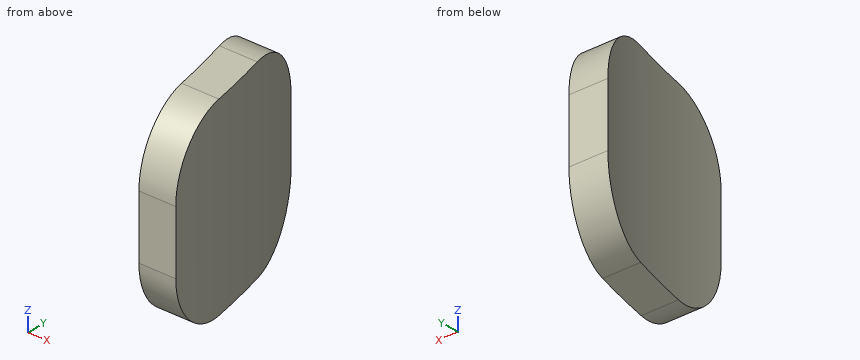
```python
from build123d import *

# Parameters (mm, degrees)
BOSS_EXTRUDE2_DEPTH     = 1066.8
CUT_EXTRUDE1_DEPTH      = 2806.00308884
CUT_EXTRUDE1_DEPTH_BACK = 2806.00308884


with BuildPart() as part:
    # Sketch1 → Boss-Extrude2 (new body)
    with BuildSketch(Plane.XY):
        with BuildLine():
            Line((1708.013552171, 1308.1), (1818.71626935, 1308.1))
            ThreePointArc((1818.71626935, 1308.1), (2198.04838822, 432.940829033), (2178.927715276, -520.7))
            Line((2178.927715276, -520.7), (2087.416444891, -520.7))
            ThreePointArc((2087.416444891, -520.7), (2106.525474721, 437.019826496), (1708.013552171, 1308.1))
        make_face()
    extrude(amount=BOSS_EXTRUDE2_DEPTH)

    # Sketch2 → Cut-Extrude1 (cut, two sides: drawn at the far end of the back side and taken through both)
    with BuildSketch(Plane(origin=(0, 0, 0), x_dir=(0, 0, -1), z_dir=(1, 0, 0)).offset(-CUT_EXTRUDE1_DEPTH_BACK)):
        with BuildLine():
            Line((-6736.08, -5778.5), (5669.28, -5778.5))
            ThreePointArc((5669.28, -5778.5), (5755.490458762, -5742.790458762), (5791.2, -5656.58))
            Line((5791.2, -5656.58), (5791.2, 6748.78))
            ThreePointArc((5791.2, 6748.78), (5755.490458762, 6834.990458762), (5669.28, 6870.7))
            Line((5669.28, 6870.7), (-6736.08, 6870.7))
            ThreePointArc((-6736.08, 6870.7), (-6822.290458762, 6834.990458762), (-6858, 6748.78))
            Line((-6858, 6748.78), (-6858, -5656.58))
            ThreePointArc((-6858, -5656.58), (-6822.290458762, -5742.790458762), (-6736.08, -5778.5))
        make_face()
        with BuildLine():
            Line((-609.6, 317.5), (-457.2, 317.5))
            ThreePointArc((-457.2, 317.5), (-349.436926547, 362.136926547), (-304.8, 469.9))
            Line((-304.8, 469.9), (-304.8, 622.3))
            ThreePointArc((-304.8, 622.3), (-349.436926547, 730.063073453), (-457.2, 774.7))
            Line((-457.2, 774.7), (-609.6, 774.7))
            ThreePointArc((-609.6, 774.7), (-717.363073453, 730.063073453), (-762, 622.3))
            Line((-762, 622.3), (-762, 469.9))
            ThreePointArc((-762, 469.9), (-717.363073453, 362.136926547), (-609.6, 317.5))
        make_face(mode=Mode.SUBTRACT)
    extrude(amount=CUT_EXTRUDE1_DEPTH + CUT_EXTRUDE1_DEPTH_BACK, mode=Mode.SUBTRACT)


solid = part.part
```
Could you check a few things on this model? Use its own coordinates, in mm. Give positions to 0.01 mm unless a question says otherwise; leave off trailing zeros. Write each loop counter-clockwise with the first axis right and the second up, starting at its lowest first coordinate (ties: lowest second). Pieces come first, ordered by that corner, then holes. Notation, with made-up numbers: (86.25, 28.5) - (109.25, 28.5) arc R5 cw to (109.25, 35.5) - close; hole circle Ø4 at (59.25, 64). An arc over 180 degrees is marked (long way). One line per item, written item: value. Start each with the question number.
Item 1: Imagine slicing it at B-B, the plane z = 546. List the corners of the cut face in (x, y) for me, and give its area (3 significant figures).
Item 2: I'm going to push flat-ended pins straight in: pin 1 (1.5 mm diameter, centred on y = 533, z = 634.5, fed in from +X); pin 2 (4 mm diameter, centred on y = 417.5, z = 488, fed in from +X); pin 3 (1 mm diameter, centred on y = 712.5, z = 683.5, fed in from -X). Where does each tip first touch, or does it pass through?
Item 3: Imagine slicing it at D-D, the plane x = 2078.5. List the corners of the cut face in (y, z) for me, and give its area (3 significant figures).
Item 4: Please list where these lines run through material, in increasing order: line 1 (Z direction, x = 2152, y = 466.5); line 2 (X direction, y = 442.5, z = 537); line 3 (Z direction, x = 2164, y = 408.5). Write a range as from..to.
Item 5: Imagine slicing it at A-A, the plane x = 2141.5. List the corners of the cut face in (y, z) for me, and give its area (3 significant figures).
Item 6: Imagine slicing it at C-C, the plane y = 715. List the corners of the cut face in (x, z) for me, and give its area (3 significant figures).
Geometry says:
1. outline: (2007.06, 774.7) arc R2151.38 cw to (2127.82, 317.5) - (2217.67, 317.5) arc R2240.28 ccw to (2102.07, 774.7) - close
1. area: 42,100 mm^2
2. pin 1: x = 2176.14
2. pin 2: x = 2201.41
2. pin 3: x = 2029.79
3. outline: (555.22, 304.8) - (622.3, 304.8) arc R152.4 ccw to (774.7, 457.2) - (774.7, 609.6) arc R152.4 ccw to (622.3, 762) - (555.22, 762) - close
3. area: 90,400 mm^2
4. line 1: 304.84..761.96
4. line 2: 2105.38..2196.14
4. line 3: 317.72..749.08
5. outline: (317.5, 457.2) arc R152.4 ccw to (469.9, 304.8) - (622.3, 304.8) arc R152.4 ccw to (657.9, 309.02) - (657.9, 757.78) arc R152.4 ccw to (622.3, 762) - (469.9, 762) arc R152.4 ccw to (317.5, 609.6) - close
5. area: 146,000 mm^2
6. outline: (2029.09, 336.24) - (2123.12, 336.24) - (2123.12, 730.56) - (2029.09, 730.56) - close
6. area: 37,100 mm^2
